Check sheet for the drawn part. Datum: minimum x, y, z corner. Units: mm. A direction names the side the tool comes from. Coordinates: 2 decimals unless noted, no trailing zeros. Loops run counter-clockwise (first coordinate to the right, second up) from the corner with the lowest first, then second, coordinate; pieces in that order, holes last.
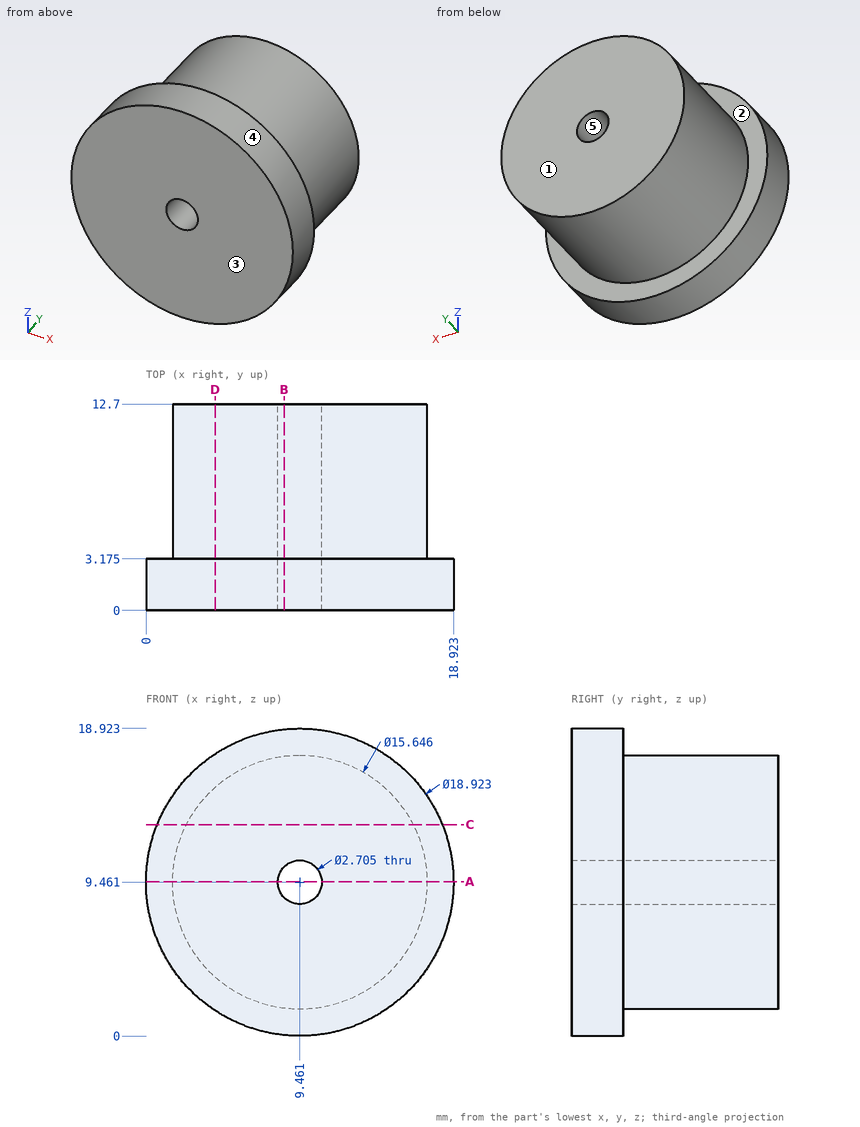
(1) Sectioned sample at C-C on z = 13. Record the cut outline in (x, y) (1 decimal), and give its area (3 significant figures).
Findings:
outline: (0.7, 0) - (18.2, 0) - (18.2, 3.2) - (16.4, 3.2) - (16.4, 12.7) - (2.5, 12.7) - (2.5, 3.2) - (0.7, 3.2) - close
area: 189 mm2
(2) Scan lines: L1, parallel to Y at x = 11.25, z = 17.25 (1 decimal); L2, parallel to Z at x = 1.25, y = 3 (1 decimal); L3, parallel to Z at x = 8, y = 6 (1 decimal). Record each from-to range of solid material in increasing order.
Findings:
L1: y = 0 to 3.2
L2: z = 4.8 to 14.2
L3: z = 1.8 to 17.1
(3) Sectioned sample at D-D on x = 4.25. Record the cut outline in (y, z) (1 decimal), and give its area (3 significant figures).
Findings:
outline: (0, 1.6) - (3.2, 1.6) - (3.2, 3.6) - (12.7, 3.6) - (12.7, 15.3) - (3.2, 15.3) - (3.2, 17.4) - (0, 17.4) - close
area: 161 mm2
(4) Sectioned sample at A-A on z = 9.5. Record the cut outline in (x, y) (1 decimal), and give its area (3 significant figures).
Findings:
outline: (0, 0) - (8.1, 0) - (8.1, 12.7) - (1.6, 12.7) - (1.6, 3.2) - (0, 3.2) - close; (10.8, 0) - (18.9, 0) - (18.9, 3.2) - (17.3, 3.2) - (17.3, 12.7) - (10.8, 12.7) - close
area: 175 mm2
(5) Draft check along X on the marked faces 3, 4 and 5. Enter one of: +X half, -X half, draft (parallel to the pull), parting line (faces both ways), or undercut.
Findings:
face 3: draft
face 4: parting line
face 5: undercut
(6) Access from +Z, -Z, +X, -X, +Y, -Y to the whole of each face (thin tool, end or side, straight path). Record for the marked faces 1 and 2.
Findings:
face 1: +Z, -Z, +X, -X, +Y
face 2: +Y
(7) Gauge pin test, flat ends, axial feed: pin 1 Ø2 at (x, y) = (13, 2.5) entering from -Z; pin 2 Ø4 at (y, z) = (8, 11.5) entering from -X; pin 3 Ø1 at (x, y) = (15, 11) entering from +Z (1 decimal). Record the tip position at first contact, or that the pin passes through.
Findings:
pin 1: stops at z = 0.35
pin 2: stops at x = 1.64
pin 3: stops at z = 15.4
(8) Sectioned sample at B-B on x = 8.5. Record the cut outline in (y, z) (1 decimal).
Findings:
outline: (0, 0) - (3.2, 0) - (3.2, 1.7) - (12.7, 1.7) - (12.7, 8.5) - (0, 8.5) - close; (0, 10.4) - (12.7, 10.4) - (12.7, 17.2) - (3.2, 17.2) - (3.2, 18.9) - (0, 18.9) - close
